Here's how the part is built. I have some questions about the finished solid (model axes, mm). A direction names the side the tool comes from. Coordinates: 2 decimals unless noted, no trailing zeros. Write each loop counter-clockwise with the first axis right and the second up, starting at its lowest first coordinate (ties: lowest second). Pieces come first, ordered by that corner, then holes. Notation, with made-up numbers: M -14.75,22 L 8.25,22 A23 ccw 8.25,31 Z; hole C 46,72 d5. An arc over 180 degrees is marked long. Use a Markdown table: item, result.
Autodesk Inventor part; units mm, degrees
ref_plane "YZ Plane" through (0, 0, 0) normal (1, 0, 0) x (0, 1, 0)
ref_plane "XZ Plane" through (0, 0, 0) normal (0, 1, 0) x (-1, 0, 0)
ref_plane "XY Plane" through (0, 0, 0) normal (0, 0, 1) x (1, 0, 0)
sketch "Sketch1" plane through (0, 0, 0) normal (0, 1, 0) x (-1, 0, 0)
  circle A0 centre (0, 0) radius 4
  dimension "d0" = 8
extrude "Extrusion1" add sketch "Sketch1" along normal blind 3
sketch "Sketch2" plane through (0, 3, 0) normal (0, 1, 0) x (1, 0, 0)
  line L0 (-1.61, -1.61) -> (1.61, -1.61)
  line L1 (1.61, -1.61) -> (1.61, 1.61)
  line L2 (1.61, 1.61) -> (-1.61, 1.61)
  line L3 (-1.61, 1.61) -> (-1.61, -1.61)
  point P0 (0, 0)
  dimension "d3" = 3.22
  dimension "d4" = 1.61
  dimension "d6" = 1.61
extrude "Extrusion2" cut sketch "Sketch2" against normal blind 1.5
properties part number "Wheel_cap"
1. Suppose I cut it at C-C on y = 2.6. Write out the boundary of the cut face in (x, z), and give its area (3 significant figures).
Answers follow:
| item | result |
|---|---|
| outline | C 0,0 d8; hole M -1.61,-1.61 L 1.61,-1.61 L 1.61,1.61 L -1.61,1.61 Z |
| area | 39.9 mm2 |
2. Suppose I cut it at A-A on x = 0. Write out the boundary of the cut face in (y, z).
Answers follow:
| item | result |
|---|---|
| outline | M 0,-4 L 3,-4 L 3,-1.61 L 1.5,-1.61 L 1.5,1.61 L 3,1.61 L 3,4 L 0,4 Z |
3. Which directions (+Z, -Z, +X, -X, +Y, -Y) give clear straight access to the entire face, cutting with the end or side of a thin tool? Please do faces 1 (the face through (0, 2, -1.61)), 2 (the face through (-2, 3, 0)).
Answers follow:
| item | result |
|---|---|
| face 1 | +Y |
| face 2 | +Z, -Z, +X, -X, +Y |
4. Suppose I cut it at D-D on y = 0.6. Write out the boundary of the cut face in (x, z), and give its area (3 significant figures).
Answers follow:
| item | result |
|---|---|
| outline | C 0,0 d8 |
| area | 50.3 mm2 |
5. I need wall thicknesses on probe 1 along Z at (x, y) = (1.5, 1.6); probe 2 along Y at (x, z) = (1, -0.5); probe 3 along X at (y, z) = (2.1, -3.25). Which ranges of each line are inside material? Lowest first, please.
Answers follow:
| item | result |
|---|---|
| probe 1 | z = -3.71 to -1.61, 1.61 to 3.71 |
| probe 2 | y = 0 to 1.5 |
| probe 3 | x = -2.33 to 2.33 |
6. Suppose I cut it at B-B on z = 0. Write out the boundary of the cut face in (x, y), and give its area (3 significant figures).
Answers follow:
| item | result |
|---|---|
| outline | M -4,0 L 4,0 L 4,3 L 1.61,3 L 1.61,1.5 L -1.61,1.5 L -1.61,3 L -4,3 Z |
| area | 19.2 mm2 |
7. We'd pull the mould along Z, two halves only. Please class faces 3 (the face through (0, 0, 0)), 4 (the face through (0, 1.5, 0)), 5 (the face through (0.867, 1.479, 3.905)): +Z half, -Z half, draft (parallel to the pull), parting line (faces both ways), or undercut.
Answers follow:
| item | result |
|---|---|
| face 3 | draft |
| face 4 | undercut |
| face 5 | parting line |
8. Will this pin go through, and if not, where does the flat tip stop? pin 1 Ø1 at (x, y) = (2.5, 0.5) entering from +Z.
Answers follow:
| item | result |
|---|---|
| pin 1 | stops at z = 3.46 |
